Autodesk Inventor part; units mm, degrees
ref_plane "Work Plane1" through (0, 0, 32.8) normal (0, 0, 1) x (1, 0, 0)
ref_plane "YZ Plane" through (0, 0, 0) normal (1, 0, 0) x (0, 1, 0)
ref_plane "XZ Plane" through (0, 0, 0) normal (0, 1, 0) x (-1, 0, 0)
sketch "Sketch1" plane through (0, 0, 0) normal (0, 0, 1) x (1, 0, 0)
  arc A0 (5.6974, 0.1712) -> (4.4165, -3.6034) centre (0, 0) ccw
  line L0 (37.7409, -2.5) -> (6.7409, -2.5)
  arc A1 (3.6983, 0.1111) -> (2.8668, -2.3391) centre (0, 0) ccw
  line L1 (6.7409, -0.5) -> (37.7409, -0.5)
  line L2 (37.7409, -0.5) -> (37.7409, -2.5)
  arc A2 (6.7409, -2.5) -> (4.4165, -3.6034) centre (6.7409, -5.5) ccw
  arc A3 (6.7409, -0.5) -> (2.8668, -2.3391) centre (6.7409, -5.5) ccw
  line L3 (3.6983, 0.1111) -> (5.6974, 0.1712)
  point P0 (5.1225, -2.5)
  dimension "d0" = 11.4
  dimension "d1" = 2
  dimension "d2" = 3
  dimension "d3" = 5
  dimension "d4" = 2
  dimension "d5" = 31
  dimension "d8" = 0.5
  dimension "d9" = 0.7
extrude "Extrusion1" add sketch "Sketch1" along normal mid plane 101.6
ref_plane "Work Plane1" through (0, 0, 32.8) normal (0, 0, 1) x (1, 0, 0)
sketch "Sketch2" plane through (0, 0, 32.8) normal (0, 0, 1) x (1, 0, 0)
  arc A0 (6.7409, -2.5) -> (4.4165, -3.6034) centre (6.7409, -5.5) ccw
  arc A1 (5.6974, 0.1712) -> (4.4165, -3.6034) centre (0, 0) ccw
  line L0 (5.6974, 0.1712) -> (3.6983, 0.1111)
  arc A2 (3.6983, 0.1111) -> (2.8668, -2.3391) centre (0, 0) ccw
  arc A3 (6.7409, -0.5) -> (2.8668, -2.3391) centre (6.7409, -5.5) ccw
  line L1 (6.7409, -0.5) -> (37.7409, -0.5) construction
  line L2 (37.7409, -0.5) -> (37.7409, -2.5) construction
  line L3 (37.7409, -2.5) -> (6.7409, -2.5) construction
  line L4 (6.7409, -0.5) -> (6.7409, -2.5)
extrude "Extrusion2" cut sketch "Sketch2" against normal blind 23.8
mirror "Mirror1" about plane through (0, 0, 0) normal (0, 0, 1) of "Extrusion2"
equation "\"d1\" = d4"
equation "\"d3\" = d2 + d4"
properties part number "HINGE PLATE 1" material "Stainless Steel"
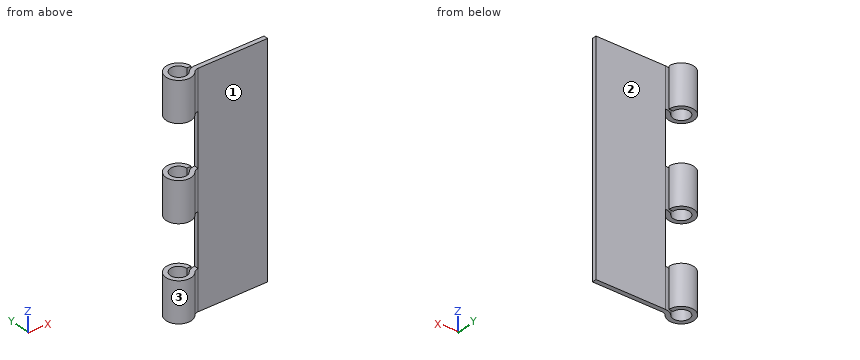
Can you work these out from the model? Positions are in its coordinate system, mm. Face numbers are marked on the shaded views. A direction names the side the tool comes from. Coordinates: 2 decimals unless noted, no trailing zeros. Loops run counter-clockwise (first coordinate to the right, second up) from the corner with the lowest first, then second, coordinate; pieces in that order, holes last. Notation, with made-up numbers: M 21,89.5 L 53,89.5 A26 cw 53,118.5 Z; hole C 60,32.5 d7. An arc over 180 degrees is marked long. Answer as CSV lines item,"result". Start each with the question number.
1. Suppose I cut it at A-A, the plane y = 2.25. List the corners of the cut face in (x, z) for me, plus the area to 3 significant figures.
2. If I drill on probe 1 along Z at (x, y) = (5, 2); probe 2 along X at (y, z) = (0.25, -1.5); probe 3 along Y at (x, z) = (22.5, -11), over which ranges is the centre line in solid material (lowest first)? Write a range as [from, to].
3. For the marked faces 1, 2 and 3, which set-ups out of +Z, -Z, +X, -X, +Y, -Y let a thin tool reach every point of the face, with its end or its side?
4. For pin 1 Ø3 at (x, z) = (23.5, 31.5) entering from -Y; pin 2 Ø2 at (y, z) = (-1, -20.5) entering from -X; pin 3 Ø9.5 at (x, z) = (20.5, -21.5) entering from +Y, each with a flat end and sliding along its axis, tell me the tip position at first contact or that it passes through.
5. Suppose I cut it at C-C, the plane x = 25. List the corners of the cut face in (y, z) for me.
6. Suppose I cut it at D-D, the plane z = 21. List the corners of the cut face in (x, y) for me, plus the area to 3 significant figures.
7. Suppose I cut it at B-B, the plane z = -4. List the corners of the cut face in (x, y) for me.
Output:
1,outline,"M -5.24,-50.8 L -2.94,-50.8 L -2.94,-32.8 L -5.24,-32.8 Z; M -5.24,-9 L -2.94,-9 L -2.94,9 L -5.24,9 Z; M -5.24,32.8 L -2.94,32.8 L -2.94,50.8 L -5.24,50.8 Z; M 2.94,-50.8 L 5.24,-50.8 L 5.24,-32.8 L 2.94,-32.8 Z; M 2.94,-9 L 5.24,-9 L 5.24,9 L 2.94,9 Z; M 2.94,32.8 L 5.24,32.8 L 5.24,50.8 L 2.94,50.8 Z"
1,area,"248 mm^2"
2,probe 1,"z = [-50.8, -32.8], [-9, 9], [32.8, 50.8]"
2,probe 2,"x = [-5.69, -3.69], [3.69, 5.69]"
2,probe 3,"y = [-2.5, -0.5]"
3,face 1,"+Z, -Z, +X, -Y"
3,face 2,"+Z, -Z, +X, +Y"
3,face 3,"+Z, -Z"
4,pin 1,"stops at y = -2.5"
4,pin 2,"stops at x = 6.74"
4,pin 3,"stops at y = -0.5"
5,outline,"M -2.5,-50.8 L -0.5,-50.8 L -0.5,50.8 L -2.5,50.8 Z"
6,outline,"M 6.74,-2.5 L 37.74,-2.5 L 37.74,-0.5 L 6.74,-0.5 Z"
6,area,"62.0 mm^2"
7,outline,"M 2.87,-2.34 A3.7 cw long 3.7,0.11 L 5.7,0.17 A5.7 ccw long 4.42,-3.6 A3 cw 6.74,-2.5 L 37.74,-2.5 L 37.74,-0.5 L 6.74,-0.5 A5 ccw Z"
